Can you work these out from the model? Positions are in its coordinate system, mm. Give positions to 0.01 mm unless a question says otherwise; leave off trailing zeros. Order: outer loops, then holes, each group sorted by start corner. A loop starts at its lowest first (then second) coordinate and runs counter-clockwise, first axis right, second up. Notation, with made-up numbers: M 87.5,68 L 117.5,68 A35 cw 117.5,102 Z; hole C 68,-28 d1. An arc over 180 degrees is marked long. Use one line per item in the form item = value. Start each with the question number.
1. I need wall thicknesses on L1, parallel to Y at x = -20, z = 10.5; L2, parallel to X at y = -3, z = 18; L3, parallel to X at y = 1.5, z = 13. Which ranges of each line are inside material? Lowest first, please.
2. Will this pin go through, and if not, where does the flat tip stop? P1, Ø5, axis at x = -20, y = 0, coming from the -Z side.
3. I want a section at A-A, the plane y = 0. List the corners of the cut face in (x, z) for me, and give its area (3 significant figures).
4. I want a section at B-B, the plane x = -20. List the corners of the cut face in (y, z) for me, and give its area (3 significant figures).
5. I want a section at C-C, the plane z = 9.5. List the corners of the cut face in (x, y) for me.
6. We'd pull the mould along X, two halves only. Please class faces 1 (the face through (23.568, -1.479, 9.86)), 2 (the face through (0, 2, 20)), 3 (the face through (-49.417, 1, 10)): +X half, -X half, draft (parallel to the pull), parting line (faces both ways), or undercut.
```python
from build123d import *

# Parameters (mm, degrees)
F0_W        = 100
F0_H        = 30
F0_R        = 4.26836
F0_R_2      = 3.862115
F1_DEPTH    = 19.6
F1_FACE_W   = 100
F1_FACE_H   = 30
F1_FACE_R   = 4.26836
F1_FACE_R_2 = 3.862115
F2_DEPTH    = 0.4


with BuildPart() as f1:
    # F0 (on Top) → F1 (new body)
    with BuildSketch(Plane.XY):
        with Locations((0.58333, 1.309117)):
            Rectangle(F0_W, F0_H)
        with Locations((-20, 0)):
            Circle(F0_R, mode=Mode.SUBTRACT)
        with Locations((20, 0)):
            Circle(F0_R_2, mode=Mode.SUBTRACT)
    extrude(amount=F1_DEPTH)

    # F1_face (on face) → F2 (join)
    with BuildSketch(Plane(origin=(0.675962, 1.356174, 19.6), x_dir=(1, 0, 0), z_dir=(0, 0, 1))):
        with Locations((-0.092632, -0.047057)):
            Rectangle(F1_FACE_W, F1_FACE_H)
        with Locations((-20.675962, -1.356174)):
            Circle(F1_FACE_R, mode=Mode.SUBTRACT)
        with Locations((19.324038, -1.356174)):
            Circle(F1_FACE_R_2, mode=Mode.SUBTRACT)
    extrude(amount=F2_DEPTH)


solid = f1.part
```
Check result:
q1.L1 = -13.69 to -4.27, 4.27 to 16.31
q1.L2 = -49.42 to -23.04, -16.96 to 17.57, 22.43 to 50.58
q1.L3 = -49.42 to -24, -16 to 16.44, 23.56 to 50.58
q2.P1 = through
q3.outline = M -49.42,0 L -24.27,0 L -24.27,20 L -49.42,20 Z; M -15.73,0 L 16.14,0 L 16.14,20 L -15.73,20 Z; M 23.86,0 L 50.58,0 L 50.58,20 L 23.86,20 Z
q3.area = 1,670 mm2
q4.outline = M -13.69,0 L -4.27,0 L -4.27,20 L -13.69,20 Z; M 4.27,0 L 16.31,0 L 16.31,20 L 4.27,20 Z
q4.area = 429 mm2
q5.outline = M -49.42,-13.69 L 50.58,-13.69 L 50.58,16.31 L -49.42,16.31 Z; hole C -20,0 d8.54; hole C 20,0 d7.72
q6.face_1 = undercut
q6.face_2 = draft
q6.face_3 = -X half
